```python
from build123d import *

# Parameters (mm, degrees)
F0_R     = 1.27
F1_DEPTH = 177.8
F2_DEPTH = 5.08
F3_DEPTH = 182.88


with BuildPart() as f1:
    # F0 (on Front) → F1 (new body)
    with BuildSketch(Plane.XZ):
        with BuildLine():
            add(Edge.make_bspline(
                [(11.9533366035, 0), (13.3596038093, 0), (15.3156895071, 1.5418011074), (11.1239910551, 6.0402650605), (-1.0569947591, 2.6537341134), (-11.0211835916, 0)],
                knots=[0, 0, 0, 0, 0.2032023134, 0.4226681756, 1, 1, 1, 1], degree=3))
            Line((-11.0211835916, 0), (11.9533366035, 0))
        make_face()
        with Locations((0.3033857343, 1.524)):
            Circle(F0_R, mode=Mode.SUBTRACT)
        with Locations((11.7333857343, 1.524)):
            Circle(F0_R, mode=Mode.SUBTRACT)
        with Locations((0.3033857343, 1.524)):
            Circle(F0_R)
        with Locations((11.7333857343, 1.524)):
            Circle(F0_R)
    extrude(amount=F1_DEPTH)

    # F0 (on Front) → F2 (join)
    with BuildSketch(Plane.XZ):
        with Locations((11.7333857343, 1.524)):
            Circle(F0_R)
        with Locations((0.3033857343, 1.524)):
            Circle(F0_R)
    extrude(amount=-F2_DEPTH)

    # F0 (on Front) → F3 (join)
    with BuildSketch(Plane.XZ):
        with Locations((0.3033857343, 1.524)):
            Circle(F0_R)
        with Locations((11.7333857343, 1.524)):
            Circle(F0_R)
    extrude(amount=F3_DEPTH)


solid = f1.part
```
Could you check a few things on this model? Use its own coordinates, in mm. Round coordinates to 2 decimals unless told otherwise and drop trailing zeros. Answer as CSV lines item,"result".
1. For pin 1 Ø2 at (x, y) = (-4, -93) entering from +Z; pin 2 Ø5 at (x, y) = (5.5, -104.5) entering from -Z; pin 3 Ø2 at (x, y) = (-3.5, -112.5) entering from +Z; pin 4 Ø8 at (x, y) = (-1, -151.5) entering from +Z, each with a flat end and sliding along its axis, tell me the tip position at first contact or that it passes through.
Filled in:
pin 1,"stops at z = 2.11"
pin 2,"stops at z = 0"
pin 3,"stops at z = 2.23"
pin 4,"stops at z = 3.47"
2. We'd pull the mould along Z, two halves only. Please class faces 1 (the face through (5, 0, 2)), 2 (the face through (0, -88, 0)): +Z half, -Z half, draft (parallel to the pull), parting line (faces both ways), or undercut.
Filled in:
face 1,"draft"
face 2,"-Z half"
3. Please list where these lines run through material, in increasing order: line 1 along Y through (x, z) = (3.75, 3.45); line 2 along Z through (x, y) = (3.25, -151.5); line 3 along Z through (x, y) = (-5.5, -86.5). Write a range as [from, to].
Filled in:
line 1,"y = [-177.8, 0]"
line 2,"z = [0, 3.52]"
line 3,"z = [0, 1.46]"
